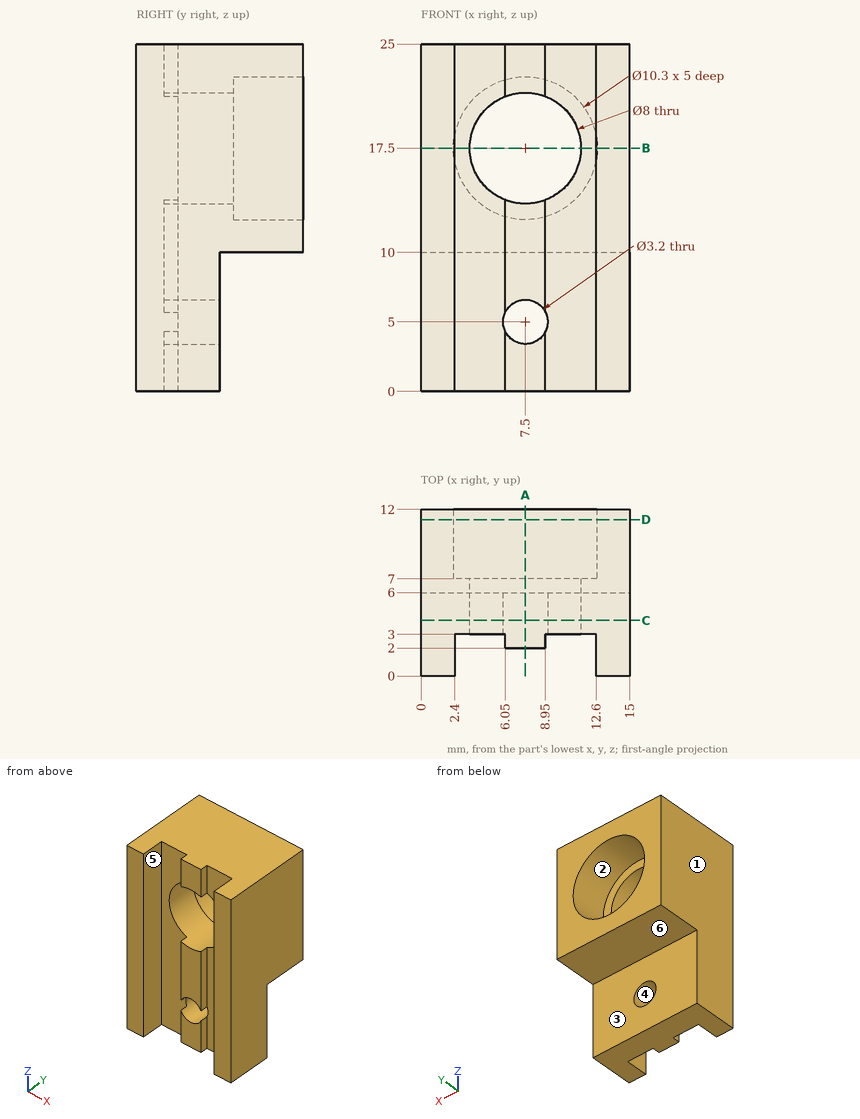
The figure shows three views and two pictorial views of one solid part (mm, origin at its lowest corner). Answer the questions. A direction names the side the tool comes from. Coordinates: 2 decimals unless noted, no trailing zeros. Loops run counter-clockwise (first coordinate to the right, second up) from the corner with the lowest first, then second, coordinate; pieces in that order, holes last. Notation, with made-up numbers: (76.25, 4.25) - (109.25, 4.25) arc R22 cw to (109.25, 36.25) - close; hole circle Ø4 at (-18, -16). An arc over 180 degrees is marked (long way). Use a Markdown table: item, result. Add a question column.
1) The mould has two halves that part along X. Classify the marked faces 1, 2 and 3: released by +X, released by -X, zero draft, split by the parting line, or undercut.
2) For the marked faces 4, 5 and 6, determine the directions among +Z, -Z, +X, -X, +Y, -Y from which every point of the face is accessible in a straight line to the end or side of a thin tool.
3) The part is cut by section C-C, the plane y = 4. Give the vertices of the cut face in (x, z).
4) Find the intervals of material crossed by line 1 (X direction, y = 2.75, z = 9.5); line 2 (Z direction, x = 6.5, y = 2.25); line 3 (X direction, y = 3.55, z = 5), in increasing order.
5) The part is cut by section A-A, the plane x = 7.5. Give the vertices of the cut face in (y, z).
6) The part is cut by section B-B, the plane z = 17.5. Give the vertices of the cut face in (x, y), and give its area (3 significant figures).
7) The part is cut by section D-D, the plane y = 11.25. Give the vertices of the cut face in (x, z), and give its area (3 significant figures).
8) Given pin 1 (3.5 mm diameter, centred on x = 7.5, z = 5, fed in from -Y); pin 2 (1 mm diameter, centred on y = 1.5, z = 21, fed in from -X); pin 3 (1.8 mm diameter, centred on x = 11, z = 13, fed in from -Y); pin 4 (1.8 mm diameter, centred on x = 8.5, y = 7.5, fed in from -Z), each flat-ended and moving along its own axis, determine where each tip first touches the part or whether it passes through.
Here are the results:
| question | item | result |
|---|---|---|
| 1 | face 1 | released by -X |
| 1 | face 2 | undercut |
| 1 | face 3 | zero draft |
| 2 | face 4 | +Y, -Y |
| 2 | face 5 | +Z, -Z, -Y |
| 2 | face 6 | -Z, +X, -X, +Y |
| 3 | outline | (0, 0) - (15, 0) - (15, 25) - (0, 25) - close; hole circle Ø8 at (7.5, 17.5); hole circle Ø3.2 at (7.5, 5) |
| 4 | line 1 | x = 0 to 2.4, 6.05 to 8.95, 12.6 to 15 |
| 4 | line 2 | z = 0 to 3.75, 6.25 to 13.63, 21.37 to 25 |
| 4 | line 3 | x = 0 to 5.9, 9.1 to 15 |
| 5 | outline | (2, 0) - (6, 0) - (6, 3.4) - (2, 3.4) - close; (2, 6.6) - (6, 6.6) - (6, 10) - (12, 10) - (12, 12.35) - (7, 12.35) - (7, 13.5) - (2, 13.5) - close; (2, 21.5) - (7, 21.5) - (7, 22.65) - (12, 22.65) - (12, 25) - (2, 25) - close |
| 6 | outline | (0, 0) - (2.4, 0) - (2.4, 3) - (3.5, 3) - (3.5, 7) - (2.35, 7) - (2.35, 12) - (0, 12) - close; (11.5, 3) - (12.6, 3) - (12.6, 0) - (15, 0) - (15, 12) - (12.65, 12) - (12.65, 7) - (11.5, 7) - close |
| 6 | area | 65.9 mm^2 |
| 7 | outline | (0, 10) - (15, 10) - (15, 25) - (0, 25) - close; hole circle Ø10.3 at (7.5, 17.5) |
| 7 | area | 142 mm^2 |
| 8 | pin 1 | stops at y = 2 |
| 8 | pin 2 | stops at x = 0 |
| 8 | pin 3 | stops at y = 3 |
| 8 | pin 4 | stops at z = 10 |
